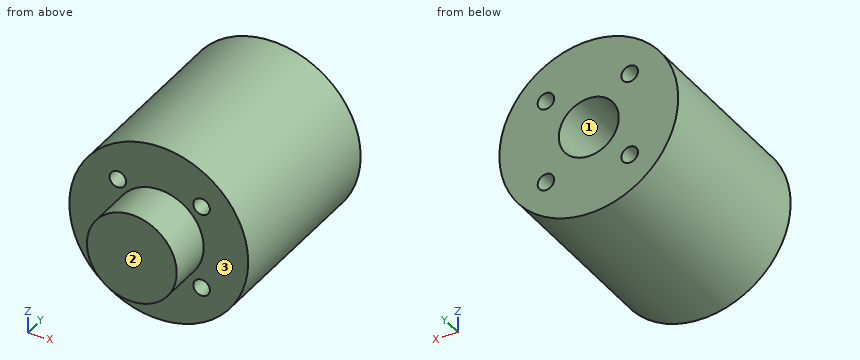
```python
from build123d import *

# Parameters (mm, degrees)
F0_R     = 11.938
F0_R_2   = 1.1049
F0_R_3   = 5.9944
F1_DEPTH = 25.4
F0_R_4   = 4.0005
F2_DEPTH = 31.496
F3_DEPTH = 31.496
F4_R     = 4.0005
F5_DEPTH = 29.21


with BuildPart() as f1:
    # F0 (on Front) → F1 (new body)
    with BuildSketch(Plane.XZ):
        Circle(F0_R)
        with Locations((-5.461991, -5.638247)):
            Circle(F0_R_2, mode=Mode.SUBTRACT)
        with Locations((5.714009, -5.638247)):
            Circle(F0_R_2, mode=Mode.SUBTRACT)
        with Locations((-5.461991, 5.537753)):
            Circle(F0_R_2, mode=Mode.SUBTRACT)
        Circle(F0_R_3, mode=Mode.SUBTRACT)
        with Locations((5.714009, 5.537753)):
            Circle(F0_R_2, mode=Mode.SUBTRACT)
    extrude(amount=F1_DEPTH)

    # F0 (on Front) → F2 (join)
    with BuildSketch(Plane.XZ):
        Circle(F0_R_3)
        Circle(F0_R_4, mode=Mode.SUBTRACT)
    extrude(amount=F2_DEPTH)

    # F0 (on Front) → F3 (join)
    with BuildSketch(Plane.XZ):
        Circle(F0_R_4)
    extrude(amount=F3_DEPTH)

    # F4 (on face) + F0 (on Front) → F5 (cut)
    with BuildSketch(Plane.XZ):
        Circle(F4_R)
    with BuildSketch(Plane.XZ):
        Circle(F0_R_4)
    extrude(amount=F5_DEPTH, mode=Mode.SUBTRACT)


solid = f1.part
```
For this review, take the finished solid that the model builds, in its own axes (mm). Face numbers are marked on the shaded views. A direction names the side the tool comes from. Round coordinates to 2 decimals unless told otherwise and drop trailing zeros. Write each loop counter-clockwise with the first axis right and the second up, starting at its lowest first coordinate (ties: lowest second). Pieces come first, ordered by that corner, then holes. Notation, with made-up numbers: (-20, -39) -> (8, -39) arc R24 ccw to (8, -20) -> close; hole circle Ø5 at (-3.5, -4.75). An arc over 180 degrees is marked (long way). One line per question, with ' | ' between items. Start each with the question number.
1) Wall thickness on line 1 along X through (y, z) = (-5, -6.5); line 2 along Z through (x, y) = (0, -23); line 3 along X through (y, z) = (-12, 5.5): over which ranges is each line inside the solid? List them lowest first.
2) Add section B-B (x = 0). Write out the cut boundary in (y, z), and give its area (3 significant figures).
3) For pin 1 Ø5 at (x, y) = (-2, -3.5) entering from +Z; pin 2 Ø5 at (x, z) = (-1.5, 8.5) entering from -Y; pin 3 Ø10 at (y, z) = (-14.5, -7.5) entering from -X; pin 4 Ø1.5 at (x, y) = (2.5, -28) entering from -Z, all flat-tipped, find the tip position at first contact; note any pin that passes through.
4) Add section D-D (x = -8). Write out the cut boundary in (y, z), and give its area (3 significant figures).
5) Add section C-C (y = -15.5). Write out the cut boundary in (x, z).
6) Machinability: for the marked faces 1, 2 and 3, which of the approach directions +Z, -Z, +X, -X, +Y, -Y give a long, thin tool a straight path to every point of the face, cutting with its end or side? Answer none if there is none.
7) Add section A-A (z = 0). Write out the cut boundary in (x, y), and give its area (3 significant figures).
Reported:
1) line 1: x = -10.01 to -6.15, -4.77 to 5.02, 6.41 to 10.01 | line 2: z = -11.94 to -4, 4 to 11.94 | line 3: x = -10.6 to -6.57, -4.36 to 4.61, 6.82 to 10.6
2) outline: (-31.5, -5.99) -> (-25.4, -5.99) -> (-25.4, -11.94) -> (0, -11.94) -> (0, -4) -> (-29.21, -4) -> (-29.21, 4) -> (0, 4) -> (0, 11.94) -> (-25.4, 11.94) -> (-25.4, 5.99) -> (-31.5, 5.99) -> close | area: 446 mm²
3) pin 1: stops at z = 11.94 | pin 2: stops at y = -25.4 | pin 3: stops at x = -11.67 | pin 4: stops at z = -5.73
4) outline: (-25.4, -8.86) -> (0, -8.86) -> (0, 8.86) -> (-25.4, 8.86) -> close | area: 450 mm²
5) outline: circle Ø23.88 at (0, 0); hole circle Ø2.21 at (-5.46, -5.64); hole circle Ø2.21 at (-5.46, 5.54); hole circle Ø8 at (0, 0); hole circle Ø2.21 at (5.71, -5.64); hole circle Ø2.21 at (5.71, 5.54)
6) face 1: +Y | face 2: +Z, -Z, +X, -X, -Y | face 3: -Y
7) outline: (-11.94, -25.4) -> (-5.99, -25.4) -> (-5.99, -31.5) -> (5.99, -31.5) -> (5.99, -25.4) -> (11.94, -25.4) -> (11.94, 0) -> (4, 0) -> (4, -29.21) -> (-4, -29.21) -> (-4, 0) -> (-11.94, 0) -> close | area: 446 mm²
